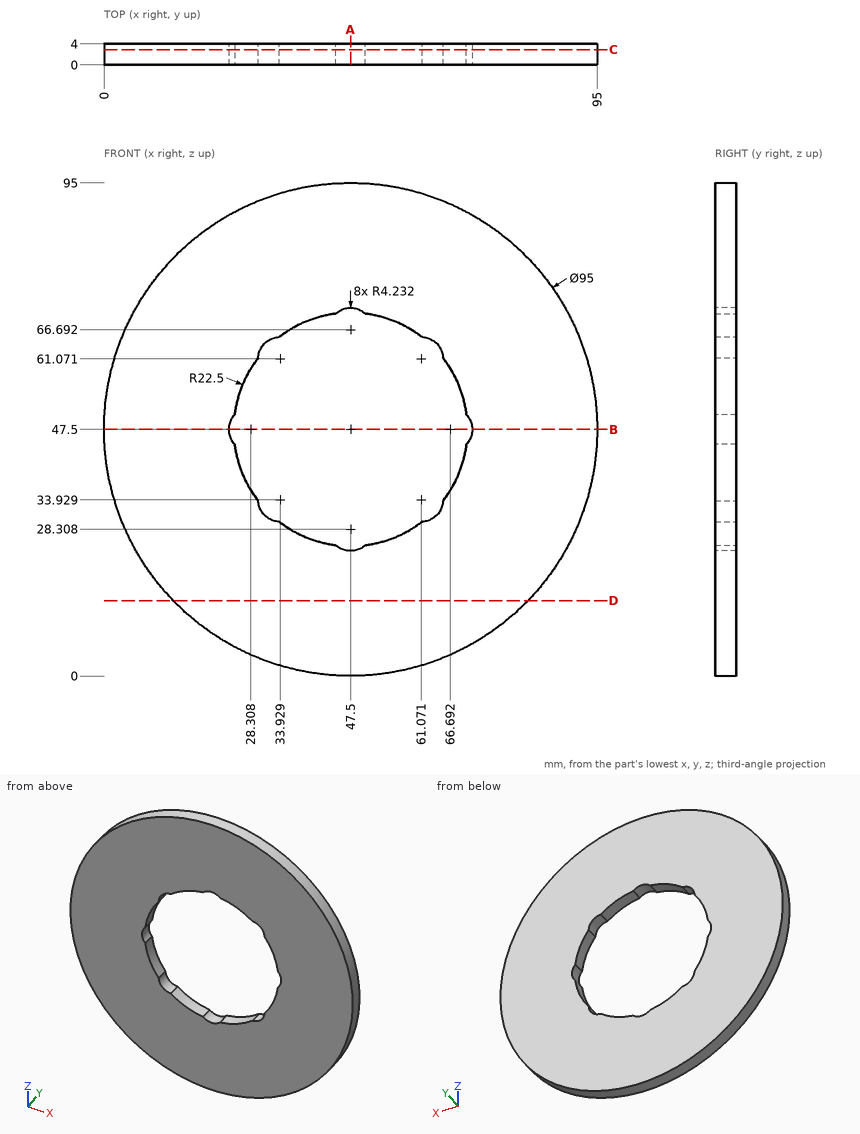
Verification items for this drawing (mm, ordinates from the low corner). Coordinates: 2 decimals unless noted, no trailing zeros. Order: outer loops, then holes, each group sorted by start corner. A loop starts at its lowest first (then second) coordinate and runs counter-clockwise, first axis right, second up. Notation, with made-up numbers: (-3, -33.5) - (46, -33.5) arc R3 cw to (46, -28.5) - close; hole circle Ø4 at (-15, -7). An arc over 180 degrees is marked (long way). Answer in a Markdown table with one row per item. Add a question column.
1. Material ranges on L1, parallel to Z at x = 44, y = 0.45 (1 decimal); L2, parallel to X at y = 3, z = 46.5 (1 decimal); L3, parallel to X at y = 1.8, z = 48 (1 decimal), recorded low to high. Write a range as [from, to].
2. Section check B-B (z = 47.5). Enter the section's corners in (x, y), plus the area to 3 significant figures.
3. Section check C-C (y = 2.9). Enter the section's corners in (x, z) (1 decimal), plus the area to 3 significant figures.
4. Section check A-A (x = 47.5). Enter the section's corners in (y, z).
5. Gauge pin test, flat ends, axial feed: pin 1 Ø4 at (x, z) = (75, 10) entering from -Y; pin 2 Ø1.5 at (y, z) = (1.5, 22) entering from +X; pin 3 Ø1.5 at (x, y) = (66, 1) entering from +Z; pin 4 Ø2 at (x, y) = (52, 0.5) entering from +Z. Record the tip position at first contact, or that the pin passes through.
6. Section check D-D (z = 14.5). Enter the section's corners in (x, y) (1 decimal).
Data:
| question | item | result |
|---|---|---|
| 1 | L1 | z = [0.1, 25.3], [69.7, 94.9] |
| 1 | L2 | x = [0, 24.2], [70.8, 95] |
| 1 | L3 | x = [0, 24.1], [70.9, 95] |
| 2 | outline | (0, 0) - (24.08, 0) - (24.08, 4) - (0, 4) - close; (70.92, 0) - (95, 0) - (95, 4) - (70.92, 4) - close |
| 2 | area | 193 mm² |
| 3 | outline | circle Ø95 at (47.5, 47.5); hole (25.2, 44.6) arc R22.5 ccw to (29.7, 33.7) arc R4.2 ccw to (33.7, 29.7) arc R22.5 ccw to (44.6, 25.2) arc R4.2 ccw to (50.4, 25.2) arc R22.5 ccw to (61.3, 29.7) arc R4.2 ccw to (65.3, 33.7) arc R22.5 ccw to (69.8, 44.6) arc R4.2 ccw to (69.8, 50.4) arc R22.5 ccw to (65.3, 61.3) arc R4.2 ccw to (61.3, 65.3) arc R22.5 ccw to (50.4, 69.8) arc R4.2 ccw to (44.6, 69.8) arc R22.5 ccw to (33.7, 65.3) arc R4.2 ccw to (29.7, 61.3) arc R22.5 ccw to (25.2, 50.4) arc R4.2 ccw to start |
| 3 | area | 5,470 mm² |
| 4 | outline | (0, 0) - (4, 0) - (4, 24.08) - (0, 24.08) - close; (0, 70.92) - (4, 70.92) - (4, 95) - (0, 95) - close |
| 5 | pin 1 | stops at y = 0 |
| 5 | pin 2 | stops at x = 88.04 |
| 5 | pin 3 | stops at z = 91.56 |
| 5 | pin 4 | stops at z = 94.87 |
| 6 | outline | (13.3, 0) - (81.7, 0) - (81.7, 4) - (13.3, 4) - close |
